from build123d import *

# Parameters (mm, degrees)
PAD_DEPTH = 23


with BuildPart() as part:
    # Sketch → Pad (new body)
    with BuildSketch(Plane.XY):
        with BuildLine():
            ThreePointArc((-63, 17), (-67.242641, 15.242641), (-69, 11))
            Line((-69, 6), (-69, 11))
            ThreePointArc((-69, 6), (-67.242641, 1.757359), (-63, 0))
            Line((-6, 0), (-63, 0))
            ThreePointArc((-6, 0), (-1.757359, 1.757359), (0, 6))
            Line((0, 11), (0, 6))
            ThreePointArc((0, 11), (-1.757359, 15.242641), (-6, 17))
            Line((-63, 17), (-6, 17))
        make_face()
        with BuildLine():
            ThreePointArc((-63, 16), (-66.535534, 14.535534), (-68, 11))
            Line((-68, 6), (-68, 11))
            ThreePointArc((-68, 6), (-66.535534, 2.464466), (-63, 1))
            Line((-6, 1), (-63, 1))
            ThreePointArc((-6, 1), (-2.464466, 2.464466), (-1, 6))
            Line((-1, 11), (-1, 6))
            ThreePointArc((-1, 11), (-2.464466, 14.535534), (-6, 16))
            Line((-63, 16), (-6, 16))
        make_face(mode=Mode.SUBTRACT)
    extrude(amount=PAD_DEPTH)


solid = part.part
The model under review builds one solid part; all positions refer to its coordinate system, in mm. A direction names the side the tool comes from. Round coordinates to 2 decimals unless told otherwise and drop trailing zeros. Loops run counter-clockwise (first coordinate to the right, second up) from the corner with the lowest first, then second, coordinate; pieces in that order, holes last. Notation, with made-up numbers: (-14, 24.5) -> (11, 24.5) arc R24 ccw to (11, 49.5) -> close; hole circle Ø11 at (54, 30.25). An arc over 180 degrees is marked (long way). Answer as CSV lines item,"result".
1) Tool access review of faces 1 (the face through (-35, 17, 11)), 2 (the face through (-2, 14, 11)): name each direction out of +Z, -Z, +X, -X, +Y, -Y from which nothing blocks a thin tool from reaching the whole face with its end or side.
Geometry results:
face 1,"+Z, -Z, +X, -X, +Y"
face 2,"+Z, -Z"
2) Add section A-A on x = -50.5. Write out the cut boundary in (y, z).
Geometry results:
outline,"(0, 0) -> (1, 0) -> (1, 23) -> (0, 23) -> close; (16, 0) -> (17, 0) -> (17, 23) -> (16, 23) -> close"
3) Draft analysis for pull direction Y (two halves, no side actions). For faces 3 (the face through (-37.2, 0.4, 23)), 4 (the face through (-67.196, 15.289, 11.339)), 5 (the face through (-67, 3, 11)), state which applies: pulls with the +Y half, pulls with the -Y half, needs draft (parallel to the pull), parting line crosses it, or undercut.
Geometry results:
face 3,"needs draft"
face 4,"pulls with the +Y half"
face 5,"undercut"
4) Add section B-B on y = 9.5. Write out the cut boundary in (x, z).
Geometry results:
outline,"(-69, 0) -> (-68, 0) -> (-68, 23) -> (-69, 23) -> close; (-1, 0) -> (0, 0) -> (0, 23) -> (-1, 23) -> close"
5) For P1, Ø2, axis at y = 14.5, z = 13, coming from the +X side; P2, Ø1, axis at x = -53, y = 14.5, coming from the -Z side; P3, Ø2, axis at y = 4.5, z = 12, coming from the +X side, all flat-tipped, find the tip position at first contact; note any pin that passes through.
Geometry results:
P1,"stops at x = -0.55"
P2,"passes through"
P3,"stops at x = -0.02"
6) To check wall thickness, follow line 1 along Y through (x, z) = (-11, 14.5); line 2 along X through (y, z) = (10, 4); line 3 along X through (y, z) = (3.25, 4). State the ranges of each line that lie inside material, in increasing order. Write a range as from..to.
Geometry results:
line 1,"y = 0..1, 16..17"
line 2,"x = -69..-68, -1..0"
line 3,"x = -68.33..-67.18, -1.82..-0.67"
7) Add section C-C on z = 7. Write out the cut boundary in (x, y).
Geometry results:
outline,"(-69, 6) arc R6 ccw to (-63, 0) -> (-6, 0) arc R6 ccw to (0, 6) -> (0, 11) arc R6 ccw to (-6, 17) -> (-63, 17) arc R6 ccw to (-69, 11) -> close; hole (-68, 6) arc R5 ccw to (-63, 1) -> (-6, 1) arc R5 ccw to (-1, 6) -> (-1, 11) arc R5 ccw to (-6, 16) -> (-63, 16) arc R5 ccw to (-68, 11) -> close"
